Geometry: see drawing. Coordinates: mm, zero at the bounding-box minimum. A direction names the side the tool comes from. Round coordinates to 2 decimals unless told otherwise and drop trailing zeros. Write each loop counter-clockwise with the first axis right and the second up, starting at its lowest first coordinate (ties: lowest second). Pieces come first, ordered by that corner, then holes. Notation, with made-up numbers: M 56,80.25 L 94,80.25 A26 cw 94,103.25 Z; hole C 59,88.5 d8. An arc over 180 degrees is marked long. Use one line per item in the form item = value. Start each with the question number.
Item 1: Section query B-B (x = 10.75). Return loops of the section in (y, z).
Item 2: Pin query (flat end, axial travel): pin 1 Ø1.5 at (x, z) = (16.5, 5) entering from -Y; pin 2 Ø1.5 at (y, z) = (2, 9.5) entering from -X. Return the tip coordinate at first contact, or that it passes through.
Item 3: Ray query, probe 1 along Y at (x, z) = (7.75, 6.5); probe 2 along X at (y, z) = (4.1, 19.25); probe 3 along X at (y, z) = (4.8, 1.75). Return the intervals inside material, ascending.
Item 4: Section query C-C (z = 7.75). Return loops of the section in (x, y).
Item 5: Reachability of the marked faces 1 and 2 from +Z, -Z, +X, -X, +Y, -Y: full face, straight path, thin tool, end or side. Return the list, or none.
Item 6: Pull-direction query (Z, two-part tool) for the marked faces 3, 4 and 5; classes: pulls with the +Z half, pulls with the -Z half, needs draft (parallel to the pull), parting line crosses it, or undercut.
Item 7: Section query A-A (z = 1.5). Return loops of the section in (x, y).
Item 8: Section query D-D (y = 2.7). Return loops of the section in (x, z).
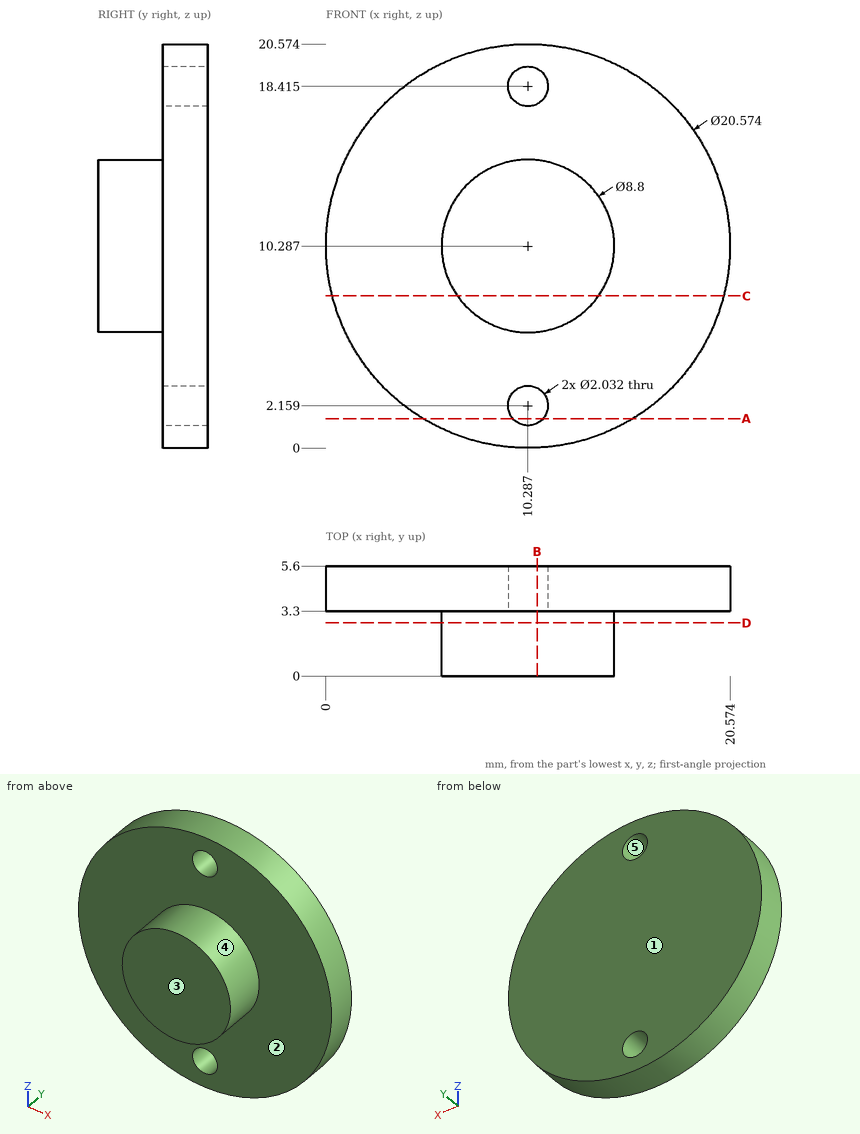
Working result:
q1.outline = M 0,5.91 L 3.3,5.91 L 3.3,3.06 L 5.6,3.06 L 5.6,17.51 L 3.3,17.51 L 3.3,14.66 L 0,14.66 Z; M 3.3,0.01 L 5.6,0.01 L 5.6,1.25 L 3.3,1.25 Z; M 3.3,19.32 L 5.6,19.32 L 5.6,20.56 L 3.3,20.56 Z
q2.pin_1 = 3.3
q2.pin_2 = 5.89
q3.probe_1 = 3.3 to 5.6
q3.probe_2 = 5.24 to 9.71, 10.87 to 15.34
q3.probe_3 = 4.55 to 9.36, 11.22 to 16.03
q4.outline = M 0.32,3.3 L 6.69,3.3 L 6.69,0 L 13.88,0 L 13.88,3.3 L 20.26,3.3 L 20.26,5.6 L 0.32,5.6 Z
q5.face_1 = +Z, -Z, +X, -X, +Y
q5.face_2 = -Y
q6.face_3 = needs draft
q6.face_4 = parting line crosses it
q6.face_5 = undercut
q7.outline = M 4.94,3.3 L 9.51,3.3 L 9.51,5.6 L 4.94,5.6 Z; M 11.06,3.3 L 15.64,3.3 L 15.64,5.6 L 11.06,5.6 Z
q8.outline = C 10.29,10.29 d8.8
